from build123d import *

# Parameters (mm, degrees)
RAMPBASE_W          = 350
RAMPBASE_H          = 350
BOSS_EXTRUDE1_DEPTH = 150
BOSS_EXTRUDE3_DEPTH = 350
BOSS_EXTRUDE5_DEPTH = 350


with BuildPart() as part:
    # rampbase → Boss-Extrude1 (new body)
    with BuildSketch(Plane(origin=(0, 0, 0), x_dir=(1, 0, 0), z_dir=(0, 1, 0))):
        Rectangle(RAMPBASE_W, RAMPBASE_H)
    extrude(amount=BOSS_EXTRUDE1_DEPTH)

    # Sketch6 → Boss-Extrude3 (add)
    with BuildSketch(Plane(origin=(175, 0, 0), x_dir=(0, 0, -1), z_dir=(1, 0, 0))):
        Polygon((-175, 150), (-175, 0), (-587, 0), align=None)
    extrude(amount=-BOSS_EXTRUDE3_DEPTH)

    # Sketch7 → Boss-Extrude5 (add)
    with BuildSketch(Plane(origin=(0, 0, -175), x_dir=(-1, 0, 0), z_dir=(0, 0, -1))):
        Polygon((175, 150), (175, 0), (587, 0), align=None)
        Polygon((-175, 0), (-587, 0), (-175, 150), align=None)
    extrude(amount=-BOSS_EXTRUDE5_DEPTH)


solid = part.part
Can you work these out from the model? Positions are in its coordinate system, mm. A direction names the side the tool comes from. Round coordinates to 2 decimals unless told otherwise and drop trailing zeros. Order: outer loops, then holes, each group sorted by start corner. A loop starts at its lowest first (then second) coordinate and runs counter-clockwise, first axis right, second up. Notation, with made-up numbers: (7, 78.5) - (44, 78.5) arc R33 cw to (44, 117.5) - close; hole circle Ø9 at (-8.75, 78). An arc over 180 degrees is marked (long way). Answer in a Markdown table with one row per item.
(1) Which directions (+Z, -Z, +X, -X, +Y, -Y) give clear straight access to the entire face, cutting with the end or side of a thin tool? Please do faces 1 (the face through (-287, 43, 175)), 2 (the face through (-2, 150, -2)), 3 (the face through (175, 43, 287)).
From the geometry:
| item | result |
|---|---|
| face 1 | +Z, -X, +Y, -Y |
| face 2 | +Z, -Z, +X, -X, +Y |
| face 3 | +Z, +X, +Y, -Y |
(2) Suppose I cut it at D-D, the plane y = 110. Please give me the cut outline in (x, z), plus the area to 3 significant figures.
From the geometry:
| item | result |
|---|---|
| outline | (-284.87, -175) - (284.87, -175) - (284.87, 175) - (175, 175) - (175, 284.87) - (-175, 284.87) - (-175, 175) - (-284.87, 175) - close |
| area | 238,000 mm2 |
(3) Suppose I cut it at B-B, the plane x = 44.5. Please give me the cut outline in (y, z).
From the geometry:
| item | result |
|---|---|
| outline | (0, -175) - (150, -175) - (150, 175) - (0, 587) - close |
(4) Suppose I cut it at A-A, the plane y = 33. Please give me the cut outline in (x, z).
From the geometry:
| item | result |
|---|---|
| outline | (-496.36, -175) - (496.36, -175) - (496.36, 175) - (175, 175) - (175, 496.36) - (-175, 496.36) - (-175, 175) - (-496.36, 175) - close |
(5) For P1, Ø6, axis at x = -34, z = 249, coming from the +Y side, with a flat end and sliding along its axis, tell me the tip position at first contact or that it passes through.
From the geometry:
| item | result |
|---|---|
| P1 | stops at y = 124.15 |
(6) Suppose I cut it at C-C, the plane z = -118. Please give me the cut outline in (x, y).
From the geometry:
| item | result |
|---|---|
| outline | (-587, 0) - (587, 0) - (175, 150) - (-175, 150) - close |
(7) Please list where these lines run through material, in increasing order: L1, parallel to X at y = 53.5, z = 265.5; L2, parallel to Y at x = 304.5, z = 134. Write a range as from..to.
From the geometry:
| item | result |
|---|---|
| L1 | x = -175..175 |
| L2 | y = 0..102.85 |
